Geometry check sheet. Reference: drawing and pictorial views, mm from the part's lowest x, y, z. A direction names the side the tool comes from. Coordinates: 2 decimals unless noted, no trailing zeros. Loops run counter-clockwise (first coordinate to the right, second up) from the corner with the lowest first, then second, coordinate; pieces in that order, holes last. Notation, with made-up numbers: (-37.5, -8) - (15.5, -8) arc R17 ccw to (15.5, 12) - close; hole circle Ø10 at (-21, 37.25). An arc over 180 degrees is marked (long way). Use a Markdown table: item, result. Add a question column.
1) Sectioned sample at D-D, the plane y = 6.75. Enter the section's corners in (x, z).
2) Sectioned sample at C-C, the plane x = 95. Enter the section's corners in (y, z).
3) Thickness scan on line 1 (Z direction, x = 12, y = 10.05); line 2 (X direction, y = 10.05, z = 4); line 3 (Z direction, x = 77, y = 3.75). Record the ranges inside material, lowest first.
4) Sectioned sample at B-B, the plane z = 19. Enter the section's corners in (x, y).
5) Tool access check on the marked faces 1, 2 and 3. Record the directions out of +Z, -Z, +X, -X, +Y, -Y that give a thin tool (end or side, any length) a straight path to the whole face; none if there is none.
6) Go/stop test with flat-tipped pins: P1, Ø4, axis at x = 45, z = 32, coming from the -Y side; P2, Ø7, axis at y = 5, z = 25.5, coming from the +X side; P3, Ø0.9, axis at y = 12, z = 18, coming from the -X side; P4, Ø2, axis at x = 12, z = 4, coming from the -Y side. Record where each tip stops, or that it passes through.
7) Sectioned sample at A-A, the plane x = 12. Enter the section's corners in (y, z).
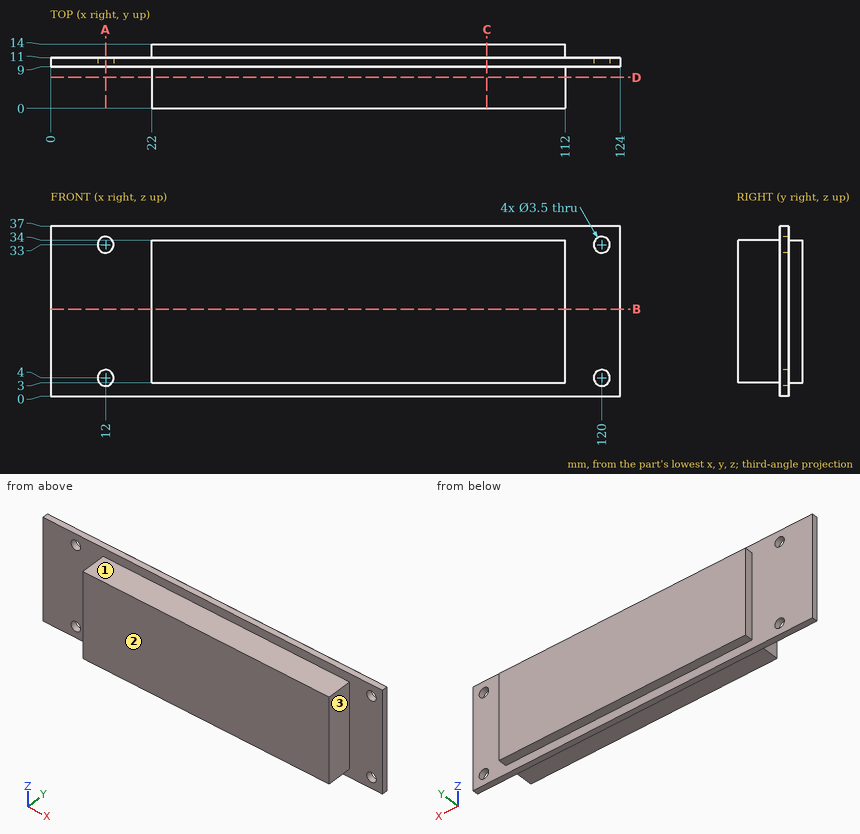
Solved:
| question | item | result |
|---|---|---|
| 1 | outline | (22, 3) - (112, 3) - (112, 34) - (22, 34) - close |
| 2 | outline | (0, 3) - (9, 3) - (9, 0) - (11, 0) - (11, 3) - (14, 3) - (14, 34) - (11, 34) - (11, 37) - (9, 37) - (9, 34) - (0, 34) - close |
| 3 | line 1 | z = 0 to 2.25, 5.75 to 31.25, 34.75 to 37 |
| 3 | line 2 | x = 0 to 10.25, 13.75 to 118.25, 121.75 to 124 |
| 3 | line 3 | z = 3 to 34 |
| 4 | outline | (0, 9) - (22, 9) - (22, 0) - (112, 0) - (112, 9) - (124, 9) - (124, 11) - (112, 11) - (112, 14) - (22, 14) - (22, 11) - (0, 11) - close |
| 5 | face 1 | +Z, +X, -X, -Y |
| 5 | face 2 | +Z, -Z, +X, -X, -Y |
| 5 | face 3 | +Z, -Z, +X, -Y |
| 6 | P1 | stops at y = 0 |
| 6 | P2 | stops at x = 112 |
| 6 | P3 | stops at x = 22 |
| 6 | P4 | passes through |
| 7 | outline | (9, 0) - (11, 0) - (11, 2.25) - (9, 2.25) - close; (9, 5.75) - (11, 5.75) - (11, 31.25) - (9, 31.25) - close; (9, 34.75) - (11, 34.75) - (11, 37) - (9, 37) - close |
